```python
from build123d import *

# Parameters (mm, degrees)
SKETCH1_R           = 1.7
BOSS_EXTRUDE1_DEPTH = 1.68656


with BuildPart() as part:
    # Sketch1 → Boss-Extrude1 (new body)
    with BuildSketch(Plane.XY):
        Polygon((0, 1), (1, 0), (110.5, 0), (111.5, 1), (111.5, 67), (110.5, 68), (104.5, 68), (103.5, 67), (103.5, 59), (100.5, 56), (11, 56), (8, 59), (8, 67), (7, 68), (1, 68), (0, 67), align=None)
        with Locations((107.5, 29.5)):
            Circle(SKETCH1_R, mode=Mode.SUBTRACT)
        with Locations((107.5, 64)):
            Circle(SKETCH1_R, mode=Mode.SUBTRACT)
        with Locations((107.5, 3.25)):
            Circle(SKETCH1_R, mode=Mode.SUBTRACT)
        with Locations((4, 64)):
            Circle(SKETCH1_R, mode=Mode.SUBTRACT)
        with Locations((4, 29.5)):
            Circle(SKETCH1_R, mode=Mode.SUBTRACT)
        with Locations((4, 3.25)):
            Circle(SKETCH1_R, mode=Mode.SUBTRACT)
    extrude(amount=BOSS_EXTRUDE1_DEPTH)


solid = part.part
```
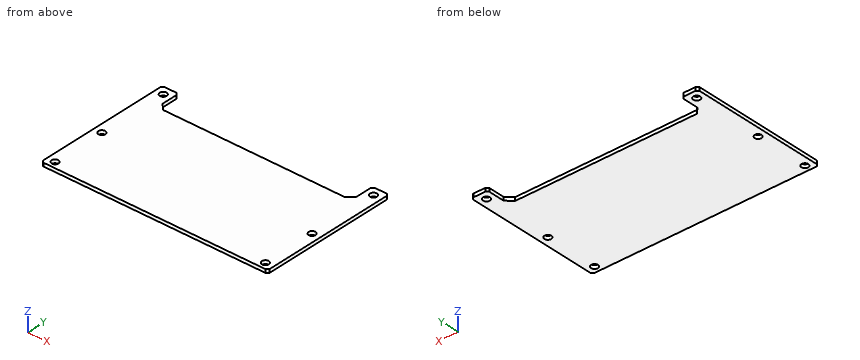
Geometry: final body of the model. Coordinates: model frame, mm. Round coordinates to 2 decimals unless told otherwise and drop trailing zeros. Write each loop counter-clockwise with the first axis right and the second up, starting at its lowest first coordinate (ties: lowest second). Pieces come first, ordered by that corner, then holes. Notation, with made-up numbers: M 83,32.25 L 98,32.25 A9 ccw 98,43.25 Z; hole C 62,-35.75 d3. An arc over 180 degrees is marked long. Answer in a Markdown table with one row per item. Add a question column.
(1) Cut plane A-A, the plane x = 107.5. Return the cut outline in (y, z), then the cut area to 3 significant figures.
(2) Ray query, L1, parallel to X at y = 64, z = 1.2; L2, parallel to X at y = 59, z = 0.75; L3, parallel to Y at x = 107.5, z = 0.85. Return the intervals inside material, ascending.
(3) Cut plane D-D, the plane y = 64. Return the cut outline in (x, z).
(4) Cut plane B-B, the plane z = 0.7. Return the cut outline in (x, y), then the cut area to 3 significant figures.
(5) Contact query for flat-ended pins moving along their axis: pin 1 (1 mm diameter, centred on x = 99.5, z = 0.5, fed in from +Y); pin 2 (4.5 mm diameter, centred on x = 4, y = 3.25, fed in from +Z). Output: stop coordinate, or through.
(6) Cut plane C-C, the plane y = 29.5. Return the cut outline in (x, z).
Established:
| question | item | result |
|---|---|---|
| 1 | outline | M 0,0 L 1.55,0 L 1.55,1.69 L 0,1.69 Z; M 4.95,0 L 27.8,0 L 27.8,1.69 L 4.95,1.69 Z; M 31.2,0 L 62.3,0 L 62.3,1.69 L 31.2,1.69 Z; M 65.7,0 L 68,0 L 68,1.69 L 65.7,1.69 Z |
| 1 | area | 97.5 mm² |
| 2 | L1 | 0 to 2.3, 5.7 to 8, 103.5 to 105.8, 109.2 to 111.5 |
| 2 | L2 | 0 to 8, 103.5 to 111.5 |
| 2 | L3 | 0 to 1.55, 4.95 to 27.8, 31.2 to 62.3, 65.7 to 68 |
| 3 | outline | M 0,0 L 2.3,0 L 2.3,1.69 L 0,1.69 Z; M 5.7,0 L 8,0 L 8,1.69 L 5.7,1.69 Z; M 103.5,0 L 105.8,0 L 105.8,1.69 L 103.5,1.69 Z; M 109.2,0 L 111.5,0 L 111.5,1.69 L 109.2,1.69 Z |
| 4 | outline | M 0,1 L 1,0 L 110.5,0 L 111.5,1 L 111.5,67 L 110.5,68 L 104.5,68 L 103.5,67 L 103.5,59 L 100.5,56 L 11,56 L 8,59 L 8,67 L 7,68 L 1,68 L 0,67 Z; hole C 4,3.25 d3.4; hole C 4,29.5 d3.4; hole C 4,64 d3.4; hole C 107.5,3.25 d3.4; hole C 107.5,29.5 d3.4; hole C 107.5,64 d3.4 |
| 4 | area | 6,390 mm² |
| 5 | pin 1 | y = 56 |
| 5 | pin 2 | z = 1.69 |
| 6 | outline | M 0,0 L 2.3,0 L 2.3,1.69 L 0,1.69 Z; M 5.7,0 L 105.8,0 L 105.8,1.69 L 5.7,1.69 Z; M 109.2,0 L 111.5,0 L 111.5,1.69 L 109.2,1.69 Z |
